from build123d import *

# Parameters (mm, degrees)
F1_DEPTH = 6.35
F2_DEPTH = 3.175
F3_SIZE  = 3.17499
F4_DEPTH = 3.175


# Not quite as in the source:
# - a fillet or chamfer is up to 0.001 mm smaller than in the source, because OpenCascade refuses the exact size


with BuildPart() as f1:
    # F0 (on Top) → F1 (new body)
    with BuildSketch(Plane.XY):
        with BuildLine():
            Line((6.1483610621, 0), (6.1483610621, 1.5875))
            ThreePointArc((6.1483610621, 1.5875), (-6.35, 0), (6.1483610621, -1.5875))
            Line((6.1483610621, -1.5875), (6.1483610621, 0))
        make_face()
        with BuildLine():
            ThreePointArc((6.1483610621, -1.5875), (6.2993885713, -0.8001272573), (6.35, 0))
            ThreePointArc((6.35, 0), (6.2993885713, 0.8001272573), (6.1483610621, 1.5875))
            Line((6.1483610621, 1.5875), (6.1483610621, 0))
            Line((6.1483610621, 0), (6.1483610621, -1.5875))
        make_face()
    extrude(amount=F1_DEPTH)

    # F0 (on Top) → F2 (join)
    with BuildSketch(Plane.XY):
        with BuildLine():
            ThreePointArc((6.1483610621, 1.5875), (6.2993885713, 0.8001272573), (6.35, 0))
            ThreePointArc((6.35, 0), (6.2993885713, -0.8001272573), (6.1483610621, -1.5875))
            Line((6.1483610621, -1.5875), (25.1983610621, -1.5875))
            ThreePointArc((25.1983610621, -1.5875), (23.6108610621, 0), (25.1983610621, 1.5875))
            Line((25.1983610621, 1.5875), (6.1483610621, 1.5875))
        make_face()
        with BuildLine():
            ThreePointArc((26.7858610621, 0), (26.3208930772, 1.1225320151), (25.1983610621, 1.5875))
            Line((25.1983610621, 1.5875), (25.1983610621, -1.5875))
            ThreePointArc((25.1983610621, -1.5875), (26.3208930772, -1.1225320151), (26.7858610621, 0))
        make_face()
        with BuildLine():
            Line((25.1983610621, -1.5875), (25.1983610621, 1.5875))
            ThreePointArc((25.1983610621, 1.5875), (23.6108610621, 0), (25.1983610621, -1.5875))
        make_face()
    extrude(amount=F2_DEPTH)

    # F3 (size 3.175 in the source; OpenCascade refuses exactly that, so slightly less here)
    f3_edges = [f1.edges().sort_by_distance(p)[0] for p in [
        (-6.148361, 1.5875, 6.35),
    ]]
    chamfer(f3_edges, length=F3_SIZE)

    # F0 (on Top) → F4 (join)
    with BuildSketch(Plane.XY):
        with BuildLine():
            ThreePointArc((26.7858610621, 0), (26.3208930772, 1.1225320151), (25.1983610621, 1.5875))
            Line((25.1983610621, 1.5875), (25.1983610621, -1.5875))
            ThreePointArc((25.1983610621, -1.5875), (26.3208930772, -1.1225320151), (26.7858610621, 0))
        make_face()
        with BuildLine():
            Line((25.1983610621, -1.5875), (25.1983610621, 1.5875))
            ThreePointArc((25.1983610621, 1.5875), (23.6108610621, 0), (25.1983610621, -1.5875))
        make_face()
    extrude(amount=-F4_DEPTH)


solid = f1.part
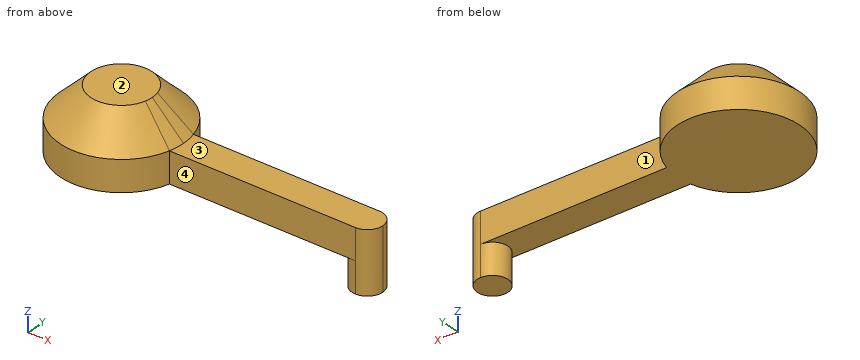
Work out the finished part from the listing and answer in its coordinate system (mm). Face numbers are marked on the shaded views. A direction names the side the tool comes from. Round coordinates to 2 decimals unless told otherwise and drop trailing zeros. Write each loop counter-clockwise with the first axis right and the second up, starting at its lowest first coordinate (ties: lowest second). Pieces come first, ordered by that corner, then holes.
1) A cutting plane is placed at D-D (x = 23). Give the vertices of the cut face in (y, z) (1 decimal).
2) Given pin 1 Ø6 at (x, y) = (17.5, -3.5) entering from +Z (3 decimals); pin 2 Ø2 at (x, z) = (-1.5, -2) entering from +Y; pin 3 Ø5 at (x, y) = (11, 2) entering from -Z; pin 4 Ø2.5 at (x, z) = (18.5, 1) entering from -Y, each flat-ended and moving along its own axis, determine where each tip first touches the part or whether it passes through.
3) Straight lines are drawn through the part: line 1 (Y direction, x = 10.5, z = 2.5); line 2 (Z direction, x = 11, y = -1.25) (3 decimals); line 3 (Z direction, x = 2, y = -0.5). For each, find the intervals that lie inside material, in ascending order.
4) A cutting plane is placed at C-C (z = -1.5). Give the vertices of the cut face in (x, y) (1 decimal), plus the area to 3 significant figures.
5) A cutting plane is placed at A-A (x = 0). Give the vertices of the cut face in (y, z) (3 decimals).
6) A tool of negligible diameter and unlimited length cuts with its end or side. For the marked faces 1, 2, 3 and 4, from which of +Z, -Z, +X, -X, +Y, -Y can it reach the whole face along a straight path? Write none if from no direction.
Completed:
1. outline: (-1.6, 0) - (1.6, 0) - (1.6, 3.2) - (-1.6, 3.2) - close
2. pin 1: stops at z = 3.175
2. pin 2: passes through
2. pin 3: stops at z = 0
2. pin 4: stops at y = -1.59
3. line 1: y = -1.59 to 1.59
3. line 2: z = 0 to 3.175
3. line 3: z = 0 to 6.35
4. outline: circle Ø3.2 at (25.2, 0)
4. area: 7.92 mm2
5. outline: (-6.35, 0) - (6.35, 0) - (6.35, 3.175) - (3.175, 6.35) - (-3.175, 6.35) - (-6.35, 3.175) - close
6. face 1: +Z, -Z, +X, +Y
6. face 2: +Z, +X, -X, +Y, -Y
6. face 3: +Z, +X, +Y, -Y
6. face 4: +Z, -Z, +X, -Y
